Verification items for this drawing (mm, ordinates from the low corner). A direction names the side the tool comes from. Round coordinates to 2 decimals unless told otherwise and drop trailing zeros. Order: outer loops, then holes, each group sorted by start corner. A loop starts at its lowest first (then second) coordinate and runs counter-clockwise, first axis right, second up. Notation, with made-up numbers: M -32,-6.5 L 13,-6.5 A17 ccw 13,26.5 Z; hole C 24.5,-6.5 d7. An arc over 180 degrees is marked long. One line per item, written item: value. Start each with the question number.
(1) Cross-section at C-C, the plane y = 49.5. Enter the section's corners in (x, z), and give its area (3 significant figures).
(2) Access from +Z, -Z, +X, -X, +Y, -Y to the whole of each face (thin tool, end or side, straight path). Record for the marked faces 1 and 2.
(3) Cross-section at B-B, the plane z = 10.5. Enter the section's corners in (x, y), and give its area (3 significant figures).
(4) Cross-section at D-D, the plane x = 23. Enter the section's corners in (y, z), and give its area (3 significant figures).
(5) Depth check by flat-ended pin: pin 1 Ø1 at (x, y) = (18.5, 12) entering from -Z; pin 2 Ø8 at (y, z) = (31.5, 15.5) entering from -X. Enter the tip coordinate at first touch or a pass-through.
(6) Cross-section at A-A, the plane x = 36.5. Enter the section's corners in (y, z).
(7) Release check for a two-part mould opening along Y. For the marked faces 3, 4, 5 and 6 record: released by +Y, released by -Y, zero draft, split by the parting line, or undercut.
(8) Thickness scan on L1, parallel to X at y = 48, z = 14.5; L2, parallel to Y at x = 36, z = 41 (1 decimal); L3, parallel to Z at x = 27, y = 57.5. Record the ranges inside material, lowest first.
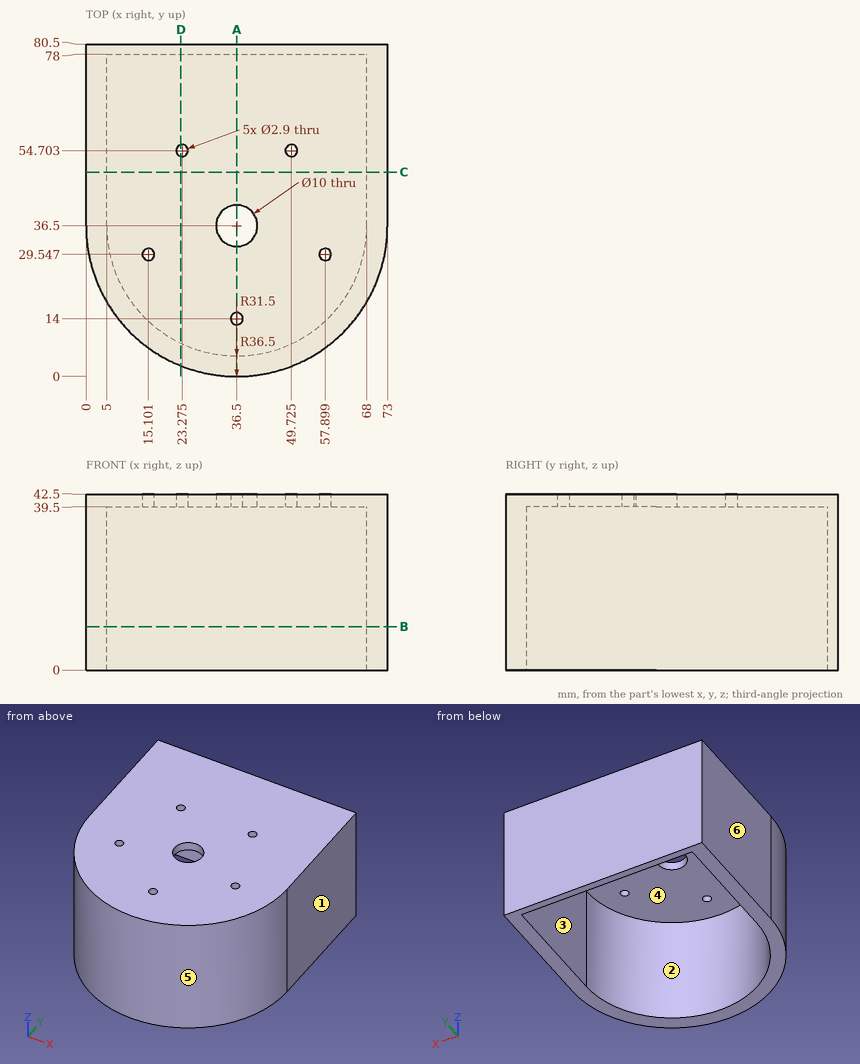
Values found:
1. outline: M 0,0 L 5,0 L 5,39.5 L 68,39.5 L 68,0 L 73,0 L 73,42.5 L 0,42.5 Z
1. area: 614 mm^2
2. face 1: +Z, -Z, +X, +Y, -Y
2. face 2: -Z
3. outline: M 0,36.5 A36.5 ccw 73,36.5 L 73,80.5 L 0,80.5 Z; hole M 5,36.5 A31.5 ccw 68,36.5 L 68,78 L 5,78 Z
3. area: 1,130 mm^2
4. outline: M 2.59,0 L 8.04,0 L 8.04,39.5 L 53.28,39.5 L 53.28,42.5 L 2.59,42.5 Z; M 56.13,39.5 L 78,39.5 L 78,0 L 80.5,0 L 80.5,42.5 L 56.13,42.5 Z
4. area: 539 mm^2
5. pin 1: z = 39.5
5. pin 2: x = 0.01
6. outline: M 0,0 L 5,0 L 5,39.5 L 12.55,39.5 L 12.55,42.5 L 0,42.5 Z; M 15.45,39.5 L 31.5,39.5 L 31.5,42.5 L 15.45,42.5 Z; M 41.5,39.5 L 78,39.5 L 78,0 L 80.5,0 L 80.5,42.5 L 41.5,42.5 Z
7. face 3: undercut
7. face 4: undercut
7. face 5: released by -Y
7. face 6: zero draft
8. L1: 0 to 5, 68 to 73
8. L2: 0 to 12.6, 15.4 to 31.5, 41.5 to 80.5
8. L3: 39.5 to 42.5
